Part model, mm, in its own coordinate system. A direction names the side the tool comes from. Coordinates: 2 decimals unless noted, no trailing zeros. Order: outer loops, then holes, each group sorted by start corner. A loop starts at its lowest first (then second) coordinate and runs counter-clockwise, first axis right, second up. Notation, with made-up numbers: (48.25, 37) - (87.25, 37) arc R22 ccw to (87.25, 59) - close; hole circle Ø5 at (-2.75, -15.5). An arc over 180 degrees is marked (long way). Use a Markdown table: item, result. Add a question column.
1) Wall check: L1, parallel to Z at x = 9.5, y = 92; L2, parallel to Y at x = 9, z = -29; L3, parallel to Z at x = 5.75, y = 91.5. Give the ranges that are in metal, low to high. Write a range as [from, to].
2) Saw through at D-D on y = 6. List the corners of the cut face in (x, z), then the cut area to 3 significant figures.
3) Saw through at C-C on z = -95. List the corners of the cut face in (x, y), then the cut area to 3 significant figures.
4) Tool access for faces 4 (the face through (7.4, 6.45, -72.43)), 5 (the face through (3.5, 14, -57.5)): list every direction of +Z, -Z, +X, -X, +Y, -Y with a clear straight run to the whole face (end or side of a thin tool).
5) Saw through at B-B on x = 4.5. Count the separate pieces of the cut face and the enclosed holes in it, then the cut area to 3 significant figures.
6) Drop flat-ended pins along their axis: P1, Ø1.8, axis at y = 6, z = -29, coming from the -X side; P2, Ø5, axis at y = 16.5, z = -53, coming from the -X side. Give the stop position or say it passes through.
7) Saw through at A-A on y = 58. List the corners of the cut face in (x, z), then the cut area to 3 significant figures.
8) Two-plate mould, pull along Z, no slides. Class faces 1 (the face through (0, 59, -38)), 2 (the face through (7, 58, -55)), 3 (the face through (7, 57, 0)): +Z half, -Z half, draft (parallel to the pull), parting line (faces both ways), or undercut.
```python
from build123d import *

# Parameters (mm, degrees)
CROQUIS1_W              = 100
CROQUIS1_H              = 116
CROQUIS1_R              = 1.5
SALIENTE_EXTRUIR1_DEPTH = 15
CROQUIS3_R              = 5
CROQUIS3_R_2            = 11
CORTAR_EXTRUIR2_DEPTH   = 7


with BuildPart() as part:
    # Croquis1 → Saliente-Extruir1 (new body)
    with BuildSketch(Plane(origin=(0, 0, 0), x_dir=(0, 0, -1), z_dir=(1, 0, 0))):
        with Locations((50, 58)):
            Rectangle(CROQUIS1_W, CROQUIS1_H)
        with Locations((5, 110)):
            Circle(CROQUIS1_R, mode=Mode.SUBTRACT)
        with Locations((29, 110)):
            Circle(CROQUIS1_R, mode=Mode.SUBTRACT)
        with Locations((5, 92)):
            Circle(CROQUIS1_R, mode=Mode.SUBTRACT)
        with Locations((29, 92)):
            Circle(CROQUIS1_R, mode=Mode.SUBTRACT)
        with Locations(Location((5, 24, 0), (0, 0, 180))):
            Circle(CROQUIS1_R, mode=Mode.SUBTRACT)
        with Locations(Location((29, 24, 0), (0, 0, 180))):
            Circle(CROQUIS1_R, mode=Mode.SUBTRACT)
        with Locations(Location((29, 6, 0), (0, 0, 180))):
            Circle(CROQUIS1_R, mode=Mode.SUBTRACT)
        with Locations(Location((5, 6, 0), (0, 0, 180))):
            Circle(CROQUIS1_R, mode=Mode.SUBTRACT)
        with Locations((31.2, 58)):
            Circle(CROQUIS1_R, mode=Mode.SUBTRACT)
        with Locations((68.8, 58)):
            Circle(CROQUIS1_R, mode=Mode.SUBTRACT)
        with Locations((71, 6)):
            Circle(CROQUIS1_R, mode=Mode.SUBTRACT)
        with Locations((95, 6)):
            Circle(CROQUIS1_R, mode=Mode.SUBTRACT)
        with Locations((95, 24)):
            Circle(CROQUIS1_R, mode=Mode.SUBTRACT)
        with Locations((71, 24)):
            Circle(CROQUIS1_R, mode=Mode.SUBTRACT)
        with Locations(Location((95, 92, 0), (0, 0, 180))):
            Circle(CROQUIS1_R, mode=Mode.SUBTRACT)
        with Locations(Location((71, 92, 0), (0, 0, 180))):
            Circle(CROQUIS1_R, mode=Mode.SUBTRACT)
        with Locations(Location((71, 110, 0), (0, 0, 180))):
            Circle(CROQUIS1_R, mode=Mode.SUBTRACT)
        with Locations(Location((95, 110, 0), (0, 0, 180))):
            Circle(CROQUIS1_R, mode=Mode.SUBTRACT)
    extrude(amount=SALIENTE_EXTRUIR1_DEPTH)

    # Croquis3 → Cortar-Extruir2 (cut)
    with BuildSketch(Plane.ZY):
        with Locations((-53.5, 99)):
            Circle(CROQUIS3_R)
        with Locations((-53.5, 17)):
            Circle(CROQUIS3_R)
        with Locations((-54.5, 58)):
            Circle(CROQUIS3_R_2)
    extrude(amount=-CORTAR_EXTRUIR2_DEPTH, mode=Mode.SUBTRACT)


solid = part.part
```
Results are:
| question | item | result |
|---|---|---|
| 1 | L1 | [-100, -96.5], [-93.5, -72.5], [-69.5, -30.5], [-27.5, -6.5], [-3.5, 0] |
| 1 | L2 | [0, 4.5], [7.5, 22.5], [25.5, 90.5], [93.5, 108.5], [111.5, 116] |
| 1 | L3 | [-100, -96.41], [-93.59, -72.41], [-69.59, -30.41], [-27.59, -6.41], [-3.59, 0] |
| 2 | outline | (0, -100) - (15, -100) - (15, -96.5) - (0, -96.5) - close; (0, -93.5) - (15, -93.5) - (15, -72.5) - (0, -72.5) - close; (0, -69.5) - (15, -69.5) - (15, -30.5) - (0, -30.5) - close; (0, -27.5) - (15, -27.5) - (15, -6.5) - (0, -6.5) - close; (0, -3.5) - (15, -3.5) - (15, 0) - (0, 0) - close |
| 2 | area | 1,320 mm2 |
| 3 | outline | (0, 0) - (15, 0) - (15, 4.5) - (0, 4.5) - close; (0, 7.5) - (15, 7.5) - (15, 22.5) - (0, 22.5) - close; (0, 25.5) - (15, 25.5) - (15, 90.5) - (0, 90.5) - close; (0, 93.5) - (15, 93.5) - (15, 108.5) - (0, 108.5) - close; (0, 111.5) - (15, 111.5) - (15, 116) - (0, 116) - close |
| 3 | area | 1,560 mm2 |
| 4 | face 4 | +X, -X |
| 4 | face 5 | -X |
| 5 | separate pieces | 1 |
| 5 | enclosed holes | 21 |
| 5 | area | 10,900 mm2 |
| 6 | P1 | through |
| 6 | P2 | x = 7 |
| 7 | outline | (0, -100) - (15, -100) - (15, -70.3) - (0, -70.3) - close; (0, -67.3) - (15, -67.3) - (15, -32.7) - (0, -32.7) - (0, -43.5) - (7, -43.5) - (7, -65.5) - (0, -65.5) - close; (0, -29.7) - (15, -29.7) - (15, 0) - (0, 0) - close |
| 7 | area | 1,260 mm2 |
| 8 | face 1 | draft |
| 8 | face 2 | undercut |
| 8 | face 3 | +Z half |
